```python
from build123d import *

# Parameters (mm, degrees)
F0_W     = 17.5
F0_H     = 23
F1_DEPTH = 240
F0_W_2   = 20
F0_H_2   = 60
F2_DEPTH = 172
F0_H_3   = 110
F3_DEPTH = 100


with BuildPart() as f1:
    # F0 (on Top) → F1 (new body)
    with BuildSketch(Plane.XY):
        with Locations((-155.7525681257, -118.5)):
            Rectangle(F0_W, F0_H)
        Polygon((-164.5025681257, -107), (-164.5025681257, -73), (-184.5025681257, -73), (-184.5025681257, -150), (179.8741881599, -150), (201.4974318743, -23.2607228812), (201.4974318743, 0), (181.4974318743, 0), (181.4974318743, -21.566840865), (162.9974318743, -130), (-147.0025681257, -130), (-164.5025681257, -130), align=None)
    extrude(amount=F1_DEPTH)



with BuildPart() as f1b:
    # F0 (on Top) → F1, piece 2 (new body)
    with BuildSketch(Plane.XY):
        Polygon((-164.5025681257, 37), (-164.5025681257, 150), (181.4974318743, 150), (181.4974318743, 60), (201.4974318743, 60), (201.4974318743, 170), (-184.5025681257, 170), (-184.5025681257, 37), align=None)
    extrude(amount=F1_DEPTH)


with BuildPart() as f1_1:
    add(f1.part)

    add(f1b.part)  # F2 merges F1b
    # F0 (on Top) → F2 (join)
    with BuildSketch(Plane.XY):
        with Locations((191.4974318743, 30)):
            Rectangle(F0_W_2, F0_H_2)
    extrude(amount=F2_DEPTH)

    # F0 (on Top) → F3 (join)
    with BuildSketch(Plane.XY):
        with Locations((-174.5025681257, -18)):
            Rectangle(F0_W_2, F0_H_3)
    extrude(amount=F3_DEPTH)


solid = f1_1.part
```
The model under review builds one solid part; all positions refer to its coordinate system, in mm. A direction names the side the tool comes from. Round coordinates to 2 decimals unless told otherwise and drop trailing zeros. Order: outer loops, then holes, each group sorted by start corner. A loop starts at its lowest first (then second) coordinate and runs counter-clockwise, first axis right, second up. Notation, with made-up numbers: (-3.5, 41) -> (10.5, 41) arc R17 cw to (10.5, 70) -> close; hole circle Ø6 at (65.25, 88.5). An arc over 180 degrees is marked (long way). Use a Markdown table: item, result.
Q1. We need section A-A on y = 95.5. Write out the cut boundary in (x, z).
Values:
| item | result |
|---|---|
| outline | (-184.5, 0) -> (-164.5, 0) -> (-164.5, 240) -> (-184.5, 240) -> close; (181.5, 0) -> (201.5, 0) -> (201.5, 240) -> (181.5, 240) -> close |
Q2. Clearance check with flat-ended pins moving along their axes: P1, Ø10, axis at x = 188.5, y = 17.5, coming from the +Z side; P2, Ø6, axis at x = -176.5, y = -28.5, coming from the +Z side; P3, Ø7, axis at y = -121, z = 120.5, coming from the +X side. State where each tip first meets the part, or that it passes through.
Values:
| item | result |
|---|---|
| P1 | stops at z = 172 |
| P2 | stops at z = 100 |
| P3 | stops at x = 185.42 |
Q3. We need section D-D on z = 87. Write out the cut boundary in (x, y).
Values:
| item | result |
|---|---|
| outline | (-184.5, -150) -> (179.87, -150) -> (201.5, -23.26) -> (201.5, 170) -> (-184.5, 170) -> close; hole (-164.5, -107) -> (-147, -107) -> (-147, -130) -> (163, -130) -> (181.5, -21.57) -> (181.5, 150) -> (-164.5, 150) -> close |
Q4. For line 1 (Y direction, x = -79.5, z = 107.5); line 2 (X direction, y = 44.5, z = 84); line 3 (X direction, y = -22, z = 227), list the stretches that pass through material, from the lowest coordinate up.
Values:
| item | result |
|---|---|
| line 1 | y = -150 to -130, 150 to 170 |
| line 2 | x = -184.5 to -164.5, 181.5 to 201.5 |
| line 3 | x = 181.42 to 201.5 |
Q5. Tool access review of faces 1 (the flat face through (-175, 37, 169)), 2 (the flat face through (191, 30, 172)), 3 (the flat face through (192, 0, 206)), 4 (the flat face through (-147.003, -119, 118)): name each direction out of +Z, -Z, +X, -X, +Y, -Y from which nothing blocks a thin tool from reaching the whole face with its end or side.
Values:
| item | result |
|---|---|
| face 1 | +Z, -X |
| face 2 | +Z, +X |
| face 3 | +Z, +X, -X |
| face 4 | +Z, -Z |
Q6. We need section B-B on x = -40.5. Write out the cut boundary in (y, z), then the cut area to 3 significant figures.
Values:
| item | result |
|---|---|
| outline | (-150, 0) -> (-130, 0) -> (-130, 240) -> (-150, 240) -> close; (150, 0) -> (170, 0) -> (170, 240) -> (150, 240) -> close |
| area | 9,600 mm^2 |
Q7. We need section C-C on z = 180. Write out the cut boundary in (x, y), then the cut area to 3 significant figures.
Values:
| item | result |
|---|---|
| outline | (-184.5, -150) -> (179.87, -150) -> (201.5, -23.26) -> (201.5, 0) -> (181.5, 0) -> (181.5, -21.57) -> (163, -130) -> (-147, -130) -> (-147, -107) -> (-164.5, -107) -> (-164.5, -73) -> (-184.5, -73) -> close; (-184.5, 37) -> (-164.5, 37) -> (-164.5, 150) -> (181.5, 150) -> (181.5, 60) -> (201.5, 60) -> (201.5, 170) -> (-184.5, 170) -> close |
| area | 23,300 mm^2 |
